The listing builds one solid part. Answer for the finished solid, in the listing's coordinates (mm). Give positions to 0.01 mm unless a question says otherwise; leave off trailing zeros. Order: outer loops, then holes, each group sorted by start corner. A loop starts at its lowest first (then second) coordinate and runs counter-clockwise, first axis right, second up. Notation, with made-up numbers: (-1, -18.75) - (4, -18.75) arc R16 cw to (4, 0.25) - close; hole circle Ø3 at (-19, 49.5). An arc over 180 degrees is marked (long way). Write each question's results on one line, items separated by ' | '. Start each with the question number.
1. Flat-ended cylindrical pins translate along their axes: pin 1 (1 mm diameter, centred on x = -7.5, z = 3.5, fed in from +Y); pin 2 (10 mm diameter, centred on y = -43.5, z = 15, fed in from -X); pin 3 (3 mm diameter, centred on y = -17.5, z = 3, fed in from -X). Find the tip coordinate at first contact, or state that the pin passes through.
2. Section B-B (x = -40) is taken. Give the vertices of the cut face in (y, z).
3. Find the intervals of material crossed by L1, parallel to Y at x = -43, z = 15.5; L2, parallel to Y at x = -6, z = 17; L3, parallel to X at y = -42.5, z = 2.25, in increasing order.
4. Section C-C (y = -32) is taken. Give the vertices of the cut face in (x, z).
5. Section A-A (z = 18.5) is taken. Give the vertices of the cut face in (x, y).
from build123d import *

# Parameters (mm, degrees)
BOSS_EXTRUDE1_DEPTH = 20
SKETCH2_W           = 20
SKETCH2_H           = 2
BOSS_EXTRUDE2_DEPTH = 3


with BuildPart() as part:
    # Sketch1 → Boss-Extrude1 (new body)
    with BuildSketch(Plane.XY):
        with BuildLine():
            Line((-45.486032275, 0.959524002), (-45.486032275, -1.040475998))
            ThreePointArc((-45.486032275, -1.040475998), (-11.544906778, -15.099350501), (2.513967725, -49.040475998))
            Line((2.513967725, -49.040475998), (4.513967725, -49.040475998))
            ThreePointArc((4.513967725, -49.040475998), (-10.130693215, -13.685136939), (-45.486032275, 0.959524002))
        make_face()
    extrude(amount=BOSS_EXTRUDE1_DEPTH)

    # Sketch2 → Boss-Extrude2 (add)
    with BuildSketch(Plane.ZY.offset(45.486032275)):
        with Locations((10, -0.040475998)):
            Rectangle(SKETCH2_W, SKETCH2_H)
    extrude(amount=BOSS_EXTRUDE2_DEPTH)


solid = part.part
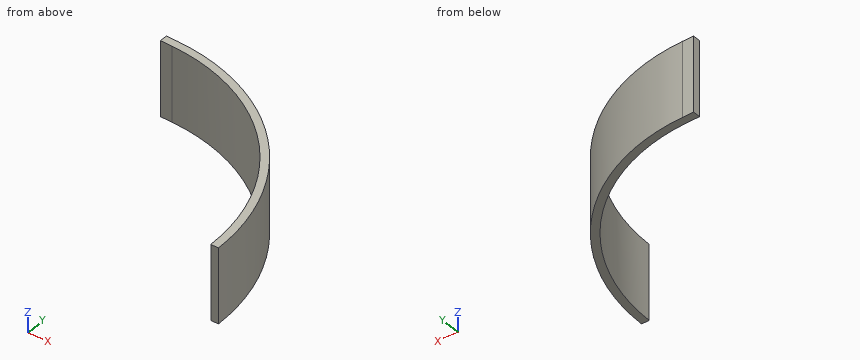
Reported:
1) pin 1: y = -15.95 | pin 2: x = 1.34 | pin 3: x = -10.67
2) outline: (-1.36, 0) - (0.66, 0) - (0.66, 20) - (-1.36, 20) - close
3) L1: -1.1 to 0.9 | L2: -21.75 to -18.37 | L3: 2.07 to 4.08
4) outline: (-0.61, 0) - (1.52, 0) - (1.52, 20) - (-0.61, 20) - close
5) outline: (-48.49, -1.04) - (-45.49, -1.04) arc R48 cw to (2.51, -49.04) - (4.51, -49.04) arc R50 ccw to (-45.49, 0.96) - (-48.49, 0.96) - close
